Input: part model. Units: mm. Frame: model coordinates. A direction names the side the tool comes from. Give positions to 0.01 mm unless a question says otherwise; leave off trailing zeros. Order: outer loops, then holes, each group sorted by start corner. A loop starts at its lowest first (then second) coordinate and runs counter-clockwise, first axis right, second up. Notation, with made-up numbers: (-1, 19.25) -> (39, 19.25) arc R37 cw to (39, 55.25) -> close; hole circle Ø11 at (74.5, 55.5). An arc over 180 degrees is marked (long way). Use a Markdown table: item, result. Add a question column.
from build123d import *

# Parameters (mm, degrees)
BOSS_EXTRUDE1_DEPTH      = 2
BOSS_EXTRUDE1_DEPTH_BACK = 2
SKETCH2_W                = 2
SKETCH2_H                = 1.5
CUT_EXTRUDE1_DEPTH       = 2


with BuildPart() as part:
    # Sketch1 → Boss-Extrude1 (new, two sides: drawn at the far end of the back side and taken through both)
    with BuildSketch(Plane.XY.offset(-BOSS_EXTRUDE1_DEPTH_BACK)):
        with BuildLine():
            Line((0, 0), (20, 0))
            Line((20, 0), (20, 3.627122207))
            Line((20, 3.627122207), (16.1, 3.627122207))
            ThreePointArc((16.1, 3.627122207), (10, 7), (3.9, 3.627122207))
            Line((3.9, 3.627122207), (0, 3.627122207))
            Line((0, 3.627122207), (0, 2))
            Line((0, 2), (0, 0))
        make_face()
        with BuildLine():
            Line((5.9, 2), (5.9, 3))
            ThreePointArc((5.9, 3), (10, 5), (14.1, 3))
            Line((14.1, 3), (14.1, 2))
            Line((14.1, 2), (5.9, 2))
        make_face(mode=Mode.SUBTRACT)
    extrude(amount=BOSS_EXTRUDE1_DEPTH + BOSS_EXTRUDE1_DEPTH_BACK)

    # Sketch2 → Cut-Extrude1 (cut)
    with BuildSketch(Plane.ZY):
        with Locations((0, 0.75)):
            Rectangle(SKETCH2_W, SKETCH2_H)
    cut_extrude1 = extrude(amount=-CUT_EXTRUDE1_DEPTH, mode=Mode.SUBTRACT)

    # Mirror1: Cut-Extrude1 across plane
    add(cut_extrude1.mirror(Plane.ZY.offset(-10)), mode=Mode.SUBTRACT)


solid = part.part
Q1. First-contact query: pin 1 (2 mm diameter, centred on x = 18.5, z = 0.5, fed in from -Y); pin 2 (1.6 mm diameter, centred on y = 0.5, z = 0, fed in from -X); pin 3 (1.2 mm diameter, centred on x = 9, z = 0.5, fed in from +Y); pin 4 (1.5 mm diameter, centred on y = 5, z = 0.5, fed in from +X). Flat tips, straight axial feed; report the tip coordinate or a pass-through.
Q2. Section query D-D (x = 10.5). Return loops of the section in (y, z).
Q3. Section query A-A (y = 2.75). Return loops of the section in (x, z), plus the area to 3 significant figures.
Q4. Access query for faces 1 (the flat face through (2, 3.627, 0)), 2 (the flat face through (14.1, 2.5, 0)), 3 (the flat face through (18, 3.627, 0)), 4 (the flat face through (19, 1.5, 0)). Directions: +Z, -Z, +X, -X, +Y, -Y. A direction counts if a zero-diameter tool reaches every point of the face in a straight line with its end or side. Return the directions, or none.
Q5. Draft query along Z for faces 5 (the flat face through (10, 0, 0)), 6 (the flat face through (1, 1.5, 0)), 7 (the flat face through (10, 1, 2)). Return one class per face: +Z half, -Z half, draft (parallel to the pull), parting line (faces both ways), or undercut.
Q6. Section query B-B (z = -1.25). Return loops of the section in (x, y) (1 decimal).
Q7. Section query C-C (x = 18.75). Return loops of the section in (y, z).
Q8. Ray query, line 1 (Y direction, x = 13.75, z = -1.1); line 2 (X direction, y = 3.5, z = -1.35); line 3 (X direction, y = 4, z = -0.2). Return the intervals inside material, ascending.
Solution:
| question | item | result |
|---|---|---|
| 1 | pin 1 | stops at y = 0 |
| 1 | pin 2 | stops at x = 2 |
| 1 | pin 3 | stops at y = 6.99 |
| 1 | pin 4 | stops at x = 15.66 |
| 2 | outline | (0, -2) -> (2, -2) -> (2, 2) -> (0, 2) -> close; (4.98, -2) -> (6.98, -2) -> (6.98, 2) -> (4.98, 2) -> close |
| 3 | outline | (0, -2) -> (5.9, -2) -> (5.9, 2) -> (0, 2) -> close; (14.1, -2) -> (20, -2) -> (20, 2) -> (14.1, 2) -> close |
| 3 | area | 47.2 mm² |
| 4 | face 1 | +Z, -Z, -X, +Y |
| 4 | face 2 | +Z, -Z |
| 4 | face 3 | +Z, -Z, +X, +Y |
| 4 | face 4 | +X, -Y |
| 5 | face 5 | draft |
| 5 | face 6 | undercut |
| 5 | face 7 | +Z half |
| 6 | outline | (0, 0) -> (20, 0) -> (20, 3.6) -> (16.1, 3.6) arc R7.2 ccw to (3.9, 3.6) -> (0, 3.6) -> close; hole (5.9, 2) -> (14.1, 2) -> (14.1, 3) arc R5.2 ccw to (5.9, 3) -> close |
| 7 | outline | (0, -2) -> (3.63, -2) -> (3.63, 2) -> (0, 2) -> (0, 1) -> (1.5, 1) -> (1.5, -1) -> (0, -1) -> close |
| 8 | line 1 | y = 0 to 2, 3.4 to 5.95 |
| 8 | line 2 | x = 0 to 6.35, 13.65 to 20 |
| 8 | line 3 | x = 4.15 to 6.93, 13.07 to 15.85 |
